Print and shaded views of the part. All mm, measured from the part's lowest x, y and z. Round coordinates to 2 decimals unless told otherwise and drop trailing zeros. Loops run counter-clockwise (first coordinate to the right, second up) from the corner with the lowest first, then second, coordinate; pieces in that order, holes last. Notation, with made-up numbers: (53, -6.5) -> (59, -6.5) arc R31 ccw to (59, 22.5) -> close; hole circle Ø6 at (12.5, -11). An arc over 180 degrees is marked (long way). Use a Markdown table: item, result.
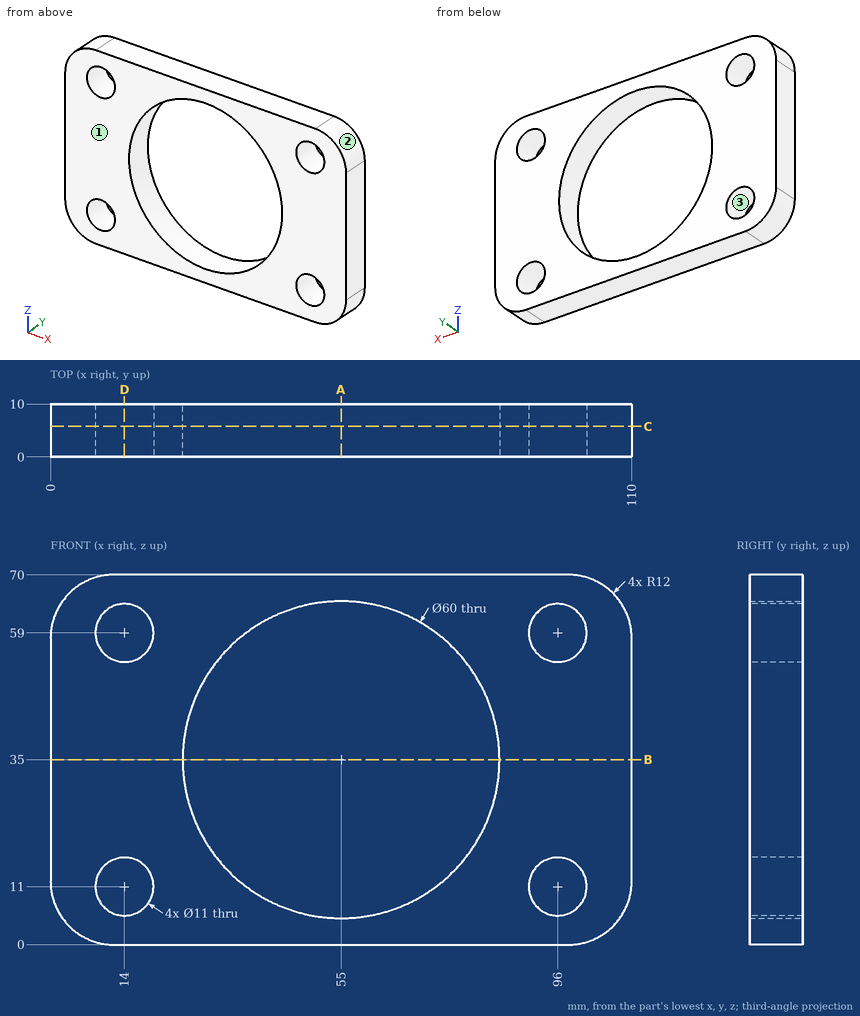
Q1. Flat gauge pins, fed straight in: pin 1 (6.5 mm diameter, centred on x = 14, z = 59, fed in from +Y); pin 2 (1.5 mm diameter, centred on x = 69, z = 8.5, fed in from +Y); pin 3 (1 mm diameter, centred on y = 5.5, z = 9, fed in from +X). Where does each tip first touch, or does it go through?
Results list:
| item | result |
|---|---|
| pin 1 | passes through |
| pin 2 | stops at y = 10 |
| pin 3 | stops at x = 109.74 |
Q2. Band-saw the part on B-B, the plane z = 35. Give the cut face in (x, y), plus the area to 3 significant figures.
Results list:
| item | result |
|---|---|
| outline | (0, 0) -> (25, 0) -> (25, 10) -> (0, 10) -> close; (85, 0) -> (110, 0) -> (110, 10) -> (85, 10) -> close |
| area | 500 mm² |
Q3. Pull direction Z, two halves, no side cores. Call the marked faces 1, 2 and 3: released by +Z, released by -Z, zero draft, split by the parting line, or undercut.
Results list:
| item | result |
|---|---|
| face 1 | zero draft |
| face 2 | released by +Z |
| face 3 | undercut |
Q4. Drill centre lines: L1, parallel to Z at x = 96, y = 8.25; L2, parallel to X at y = 3.5, z = 15.5; L3, parallel to Z at x = 55, y = 6.75. Where is each one in solid material? Low to high. Write a range as from..to.
Results list:
| item | result |
|---|---|
| L1 | z = 0..5.5, 16.5..53.5, 64.5..70 |
| L2 | x = 0..10.84, 17.16..32.2, 77.8..92.84, 99.16..110 |
| L3 | z = 0..5, 65..70 |
Q5. Band-saw the part on A-A, the plane x = 55. Give the cut face in (y, z).
Results list:
| item | result |
|---|---|
| outline | (0, 0) -> (10, 0) -> (10, 5) -> (0, 5) -> close; (0, 65) -> (10, 65) -> (10, 70) -> (0, 70) -> close |
Q6. Band-saw the part on D-D, the plane x = 14. Give the cut face in (y, z).
Results list:
| item | result |
|---|---|
| outline | (0, 0) -> (10, 0) -> (10, 5.5) -> (0, 5.5) -> close; (0, 16.5) -> (10, 16.5) -> (10, 53.5) -> (0, 53.5) -> close; (0, 64.5) -> (10, 64.5) -> (10, 70) -> (0, 70) -> close |
Q7. Band-saw the part on C-C, the plane y = 5.75. Give the cut face in (x, z).
Results list:
| item | result |
|---|---|
| outline | (0, 12) arc R12 ccw to (12, 0) -> (98, 0) arc R12 ccw to (110, 12) -> (110, 58) arc R12 ccw to (98, 70) -> (12, 70) arc R12 ccw to (0, 58) -> close; hole circle Ø11 at (14, 11); hole circle Ø11 at (14, 59); hole circle Ø60 at (55, 35); hole circle Ø11 at (96, 11); hole circle Ø11 at (96, 59) |
